Autodesk Inventor part; units mm, degrees
ref_plane "Work Plane2" through (3.35, 0, 0) normal (0, 0, -1) x (1, 0, 0)
ref_plane "YZ Plane" through (0, 0, 0) normal (1, 0, 0) x (0, 1, 0)
ref_plane "XZ Plane" through (0, 0, 0) normal (0, 1, 0) x (-1, 0, 0)
sketch "Sketch1" plane through (0, 0, 0) normal (0, 0, 1) x (1, 0, 0)
  line L0 (1.88, 0) -> (20, 0)
  line L1 (20, 0) -> (20, 2)
  line L2 (20, 2) -> (3.6, 2)
  line L3 (3.6, 2) -> (3.1706, 1.7853)
  line L4 (3.1706, 1.7853) -> (2.2, 1.7853)
  line L5 (0, 3.5) -> (0, 2.11)
  line L6 (0, 2.11) -> (1.0316, 1.5957)
  line L7 (1.0316, 1.5957) -> (1.88, 0)
  line L8 (-4, 0) -> (24, 0)
  line L9 (0, -0.7) -> (0, 4.2)
  line L10 (0, 3.5) -> (0.4853, 3.5)
  line L11 (0.4853, 3.5) -> (2.2, 1.7853)
  line L12 (3.6, 2) -> (1.9853, 2) construction
  dimension "d1" = 16.4
  dimension "d2" = 4
  dimension "d3" = 3.5706
  dimension "d4" = 4.22
  dimension "d5" = 26.5
  dimension "d6" = 62
  dimension "d7" = 1.88
  dimension "d8" = 0.4294
  dimension "d12" = 7
  dimension "d13" = 45
  dimension "d15" = 20
  dimension "d24" = 2.2
revolve "Body" add sketch "Sketch1" angle 360 about axis through (1.88, 0, 0) along (1, 0, 0) contours L7 L6 L5 L10 L11 L4 L3 L2 L1 L0
sketch "Sketch2" plane through (0, 0, 0) normal (-1, 0, 0) x (0, 0, 1)
  line L0 (0, 2.11) -> (0, 0) construction
  line L1 (0, 0) -> (2.11, 0) construction
  arc A0 (0.633, 0) -> (0, 0.633) centre (0, 0) ccw construction
  arc A1 (0.7385, 0) -> (0, 0.7385) centre (0, 0) ccw construction
  arc A2 (2.0511, 0.495) -> (0.495, 2.0511) centre (0, 0) ccw
  line L2 (0, 0) -> (1.492, 1.492) construction
  line L3 (0.495, 2.0511) -> (0.3793, 0.6337)
  line L4 (2.0511, 0.495) -> (0.6337, 0.3793)
  arc A3 (0.495, 2.0511) -> (0, 2.11) centre (0, 0) ccw
  arc A4 (2.11, 0) -> (2.0511, 0.495) centre (0, 0) ccw
  line L5 (0, -4.9) -> (0, 4.9)
  line L6 (-4.9, 0) -> (4.9, 0)
  arc A5 (0.495, -2.0511) -> (2.0511, -0.495) centre (0, 0) ccw
  line L7 (0.495, -2.0511) -> (0.3793, -0.6337)
  line L8 (2.0511, -0.495) -> (0.6337, -0.3793)
  arc A6 (0, -2.11) -> (0.495, -2.0511) centre (0, 0) ccw
  arc A7 (2.0511, -0.495) -> (2.11, 0) centre (0, 0) ccw
  arc A8 (-0.495, 2.0511) -> (-2.0511, 0.495) centre (0, 0) ccw
  line L9 (-0.495, 2.0511) -> (-0.3793, 0.6337)
  line L10 (-2.0511, 0.495) -> (-0.6337, 0.3793)
  arc A9 (0, 2.11) -> (-0.495, 2.0511) centre (0, 0) ccw
  arc A10 (-2.0511, 0.495) -> (-2.11, 0) centre (0, 0) ccw
  arc A11 (-0.495, -2.0511) -> (0, -2.11) centre (0, 0) ccw
  arc A12 (-2.0511, -0.495) -> (-0.495, -2.0511) centre (0, 0) ccw
  arc A13 (-2.11, 0) -> (-2.0511, -0.495) centre (0, 0) ccw
  line L11 (-2.0511, -0.495) -> (-0.6337, -0.3793)
  line L12 (-0.495, -2.0511) -> (-0.3793, -0.6337)
  arc A14 (0.3793, 0.6337) -> (0.6337, 0.3793) centre (0.6145, 0.6145) ccw
  arc A15 (0.6337, -0.3793) -> (0.3793, -0.6337) centre (0.6145, -0.6145) ccw
  arc A16 (-0.6337, 0.3793) -> (-0.3793, 0.6337) centre (-0.6145, 0.6145) ccw
  arc A17 (-0.3793, -0.6337) -> (-0.6337, -0.3793) centre (-0.6145, -0.6145) ccw
  point P0 (1.492, -1.492)
  point P1 (-1.492, 1.492)
  point P2 (-1.492, -1.492)
  dimension "d17" = 1.266
  dimension "d18" = 1.477
  dimension "d19" = 4.22
  dimension "d20" = 45
  dimension "d21" = 0.495
extrude "Slot" add sketch "Sketch2" against normal up to next draft 5 contours L4 A14 L3 A2 | A5 L7 A15 L8 | L9 A16 L10 A8 | A12 L11 A17 L12
fillet "Fillet1" radius 0.198 4 edges at (0, 2.11, 0) (0, 0, -2.11) (0, -2.11, 0) (0, 0, 2.11)
thread "Thread"
chamfer "Chamfer1" distance 0.4294 distance2 0.2147 1 edges at (20, -2, 0) measured on face at (20, -0.6473, 0.1595)
ref_plane "Work Plane2" through (3.35, 0, 0) normal (0, 0, -1) x (1, 0, 0)
equation "\"d17\" = 0.3 * SDM"
equation "\"d18\" = 0.35 * SDM"
equation "\"d19\" = SDM"
equation "\"d21\" = 0.5 * SBR"
equation "\"d1\" = GEL"
equation "\"d2\" = GD"
equation "\"d3\" = BDM"
equation "\"d4\" = SDM"
equation "\"d7\" = INTI"
equation "\"d8\" = GAL"
equation "\"d12\" = KOD"
equation "\"d13\" = 0.5 * SEWI"
equation "\"d15\" = NLG"
equation "\"d24\" = KOH"
equation "\"d23\" = 0.2 * SBR"
equation "\"d10\" = GEL"
equation "\"d25\" = -0.5 * SPD + 0.5 * GD"
equation "\"d26\" = 0.5 * GAL"
equation "\"NLG\" = 20"
equation "\"GEL\" = 16.4"
equation "\"GAL\" = 0.61345 * PTC"
equation "\"SPD\" = NND - 1.2269 * PTC"
equation "\"KOD\" = 7"
equation "\"KOH\" = 2.2"
equation "\"SBR\" = 0.99"
equation "\"INTI\" = 1.88"
equation "\"SDM\" = 4.22"
equation "\"GD\" = NND"
equation "\"BDM\" = NND - GAL"
equation "\"SEWI\" = 90deg"
equation "\"d9\" = SDM"
equation "\"GUL\" = 0.61345 * PTC"
equation "\"TOA\" = 30deg"
equation "\"EPV\" = 4.2"
equation "\"THREADDIA\" = 4"
equation "\"RR\" = 0.4"
equation "\"PTC\" = 0.7"
equation "\"NND\" = 4"
equation "\"GD1\" = THREADDIA - 1.2269 * PTC"
properties part number "AS 1427 - M4 x 20" material "Steel, Mild"
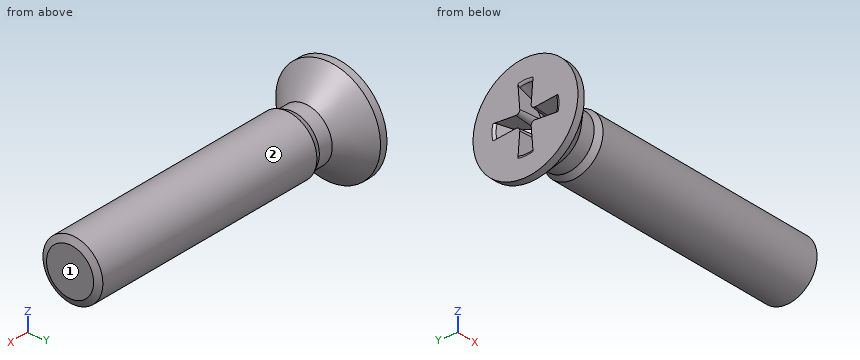
Could you check a few things on this model? Use its own coordinates, in mm. Face numbers are marked on the shaded views. A direction names the side the tool comes from. Coordinates: 2 decimals unless noted, no trailing zeros. Order: outer loops, then holes, each group sorted by start corner. A loop starts at its lowest first (then second) coordinate and runs counter-clockwise, first axis right, second up. Notation, with made-up numbers: (-0.5, -22.75) - (34.5, -22.75) arc R16 ccw to (34.5, 1.25) - close; hole circle Ø2 at (-6, -29.5). An arc over 180 degrees is marked (long way). Answer in a Markdown table with one row per item. Add a question column.
(1) I need wall thicknesses on L1, parallel to X at y = -2.5, z = -1.75; L2, parallel to Z at x = 11.75, y = 1.25; L3, parallel to X at y = -0.75, z = 2. Which ranges of each line are inside material? Lowest first, please.
(2) If we section it at A-A, the plane x = 14.75: Please give me the cut outline in (y, z), then the cut area to 3 significant figures.
(3) Will this pin go through, and if not, where does the flat tip stop? pin 1 (1.5 mm diameter, centred on x = 10.5, y = 2.5, fed in from +Z).
(4) On a 3-axis mill with a long thin cutter (end or side, diameter ignored), from which of +Z, -Z, +X, -X, +Y, -Y can I reach the whole of each face in a straight line? I mean the marked faces 1 and 2. Say none if no direction works.
Results are:
| question | item | result |
|---|---|---|
| 1 | L1 | x = 0 to 0.93 |
| 1 | L2 | z = -1.56 to 1.56 |
| 1 | L3 | x = 0 to 1.85 |
| 2 | outline | circle Ø4 at (0, 0) |
| 2 | area | 12.6 mm2 |
| 3 | pin 1 | stops at z = 0.97 |
| 4 | face 1 | +Z, -Z, +X, +Y, -Y |
| 4 | face 2 | +X |
